```python
from build123d import *

# Parameters (mm, degrees)
F0_W     = 2
F0_H     = 4
F1_DEPTH = 8
F2_DEPTH = 9
F3_T     = -2
F4_R     = 5
F5_R     = 5
F6_W     = 8.62
F6_H     = 2
F7_DEPTH = 6


with BuildPart() as f1:
    # F0 (on Top) → F1 (new body)
    with BuildSketch(Plane.XY):
        Polygon((-23.121336045, 19.3491095896), (-19.6572344299, 21.3491095896), (-20.6572344299, 23.0811603972), (-24.121336045, 21.0811603972), align=None)
        Polygon((-7.4004464167, 26.1161683716), (-26.3174884677, 15.1944090512), (-26.3174884677, 10.3491095896), (-26.3174884677, 6.6491095896), (-26.3174884677, -15.1944090512), (-22.121336045, -17.617058782), (-18.917042051, -19.467058782), (0, -30.3888181024), (4.1961524227, -27.9661683716), (7.4004464167, -26.1161683716), (26.3174884677, -15.1944090512), (26.3174884677, -10.3491095896), (26.3174884677, -6.6491095896), (26.3174884677, 15.1944090512), (22.121336045, 17.617058782), (18.917042051, 19.467058782), (0, 30.3888181024), (-4.1961524227, 27.9661683716), align=None)
        Polygon((0, -21.59), (-18.6974884677, -10.795), (-18.6974884677, 10.795), (0, 21.59), (18.6974884677, 10.795), (18.6974884677, -10.795), align=None, mode=Mode.SUBTRACT)
        Polygon((-5.1961524227, -29.6982191792), (-8.6602540378, -27.6982191792), (-9.6602540378, -29.4302699868), (-6.1961524227, -31.4302699868), align=None)
        with Locations((29.3174884677, 8.3491095896)):
            Rectangle(F0_W, F0_H)
        with Locations((-29.3174884677, -8.3491095896)):
            Rectangle(F0_W, F0_H)
        Polygon((-26.3174884677, -15.1944090512), (-26.3174884677, 6.6491095896), (-28.3174884677, 6.6491095896), (-28.3174884677, -6.3491095896), (-28.3174884677, -10.3491095896), (-28.3174884677, -16.3491095896), (-23.121336045, -19.3491095896), (-22.121336045, -17.617058782), align=None)
        Polygon((-26.3174884677, 10.3491095896), (-26.3174884677, 15.1944090512), (-7.4004464167, 26.1161683716), (-8.4004464167, 27.8482191792), (-19.6572344299, 21.3491095896), (-23.121336045, 19.3491095896), (-28.3174884677, 16.3491095896), (-28.3174884677, 10.3491095896), align=None)
        Polygon((0, -30.3888181024), (-18.917042051, -19.467058782), (-19.917042051, -21.1991095896), (-8.6602540378, -27.6982191792), (-5.1961524227, -29.6982191792), (0, -32.6982191792), (5.1961524227, -29.6982191792), (4.1961524227, -27.9661683716), align=None)
        Polygon((28.3174884677, -10.3491095896), (26.3174884677, -10.3491095896), (26.3174884677, -15.1944090512), (7.4004464167, -26.1161683716), (8.4004464167, -27.8482191792), (19.6572344299, -21.3491095896), (23.121336045, -19.3491095896), (28.3174884677, -16.3491095896), align=None)
        Polygon((23.121336045, -19.3491095896), (19.6572344299, -21.3491095896), (20.6572344299, -23.0811603972), (24.121336045, -21.0811603972), align=None)
        Polygon((-5.1961524227, 29.6982191792), (-4.1961524227, 27.9661683716), (0, 30.3888181024), (18.917042051, 19.467058782), (19.917042051, 21.1991095896), (8.6602540378, 27.6982191792), (5.1961524227, 29.6982191792), (0, 32.6982191792), align=None)
        Polygon((6.1961524227, 31.4302699868), (5.1961524227, 29.6982191792), (8.6602540378, 27.6982191792), (9.6602540378, 29.4302699868), align=None)
        Polygon((23.121336045, 19.3491095896), (22.121336045, 17.617058782), (26.3174884677, 15.1944090512), (26.3174884677, -6.6491095896), (28.3174884677, -6.6491095896), (28.3174884677, 6.3491095896), (28.3174884677, 10.3491095896), (28.3174884677, 16.3491095896), align=None)
    extrude(amount=F1_DEPTH)

    # F0 (on Top) → F2 (join)
    with BuildSketch(Plane.XY):
        Polygon((-18.6974884677, 10.795), (-18.6974884677, -10.795), (0, -21.59), (18.6974884677, -10.795), (18.6974884677, 10.795), (0, 21.59), align=None)
    extrude(amount=F2_DEPTH)

    # F3: a shell. OpenCascade refuses it in one call, so the cavity is built on its own and cut out:
    # the body offset inwards by the wall thickness, plus a prism from it out through each open face.
    f3_core = offset(f1.part, amount=F3_T, kind=Kind.INTERSECTION, mode=Mode.PRIVATE)
    f3_exits = [f3_core.faces().sort_by_distance(p)[0] for p in [
        (0, 0, 2),
    ]]
    add(f3_core, mode=Mode.SUBTRACT)
    extrude(f3_exits, amount=-F3_T, mode=Mode.SUBTRACT)

    # F4
    f4_edges = [f1.edges().sort_by_distance(p)[0] for p in [
        (-18.697488, 10.795, 8.5),
        (-18.697488, -10.795, 8.5),
        (0, -21.59, 8.5),
        (18.697488, -10.795, 8.5),
        (18.697488, 10.795, 8.5),
        (0, 21.59, 8.5),
    ]]
    fillet(f4_edges, radius=F4_R)

    # F5
    f5_edges = [f1.edges().sort_by_distance(p)[0] for p in [
        (16.697488, -9.640299, 6.5),
        (0, -19.280599, 6.5),
        (-16.697488, -9.640299, 6.5),
        (-16.697488, 9.640299, 6.5),
        (0, 19.280599, 6.5),
        (16.697488, 9.640299, 6.5),
    ]]
    fillet(f5_edges, radius=F5_R)

    # F6 (on face) → F7 (join)
    with BuildSketch(Plane(origin=(0, 0, 6), x_dir=(1, 0, 0), z_dir=(0, 0, -1))):
        Polygon((15.2029661558, 21.6113814999), (13.4611243361, 22.6170343434), (8.3950167715, 15.6640247696), (10.0114517622, 14.4862565748), align=None)
        with Locations((-22.0074884677, 4.1833669636)):
            Rectangle(F6_W, F6_H)
        with Locations((22.0074884677, -0.0066501563)):
            Rectangle(F6_W, F6_H)
        Polygon((-12.5819755408, -13.1710924962), (-16.8919755408, -20.6362314769), (-15.1599247332, -21.6362314769), (-10.8499247332, -14.1710924962), align=None)
    extrude(amount=F7_DEPTH)


solid = f1.part
```
Geometry: final body of the model. Coordinates: model frame, mm. A direction names the side the tool comes from. Round coordinates to 2 decimals unless told otherwise and drop trailing zeros. Order: outer loops, then holes, each group sorted by start corner. A loop starts at its lowest first (then second) coordinate and runs counter-clockwise, first axis right, second up. Notation, with made-up numbers: (-20, 50.25) - (38, 50.25) arc R20 ccw to (38, 66.25) - close; hole circle Ø1 at (-4.75, -19). An arc over 180 degrees is marked (long way). Write item = value, one per line. Start each with the question number.
Q1. Cut plane A-A on y = 3. Return the cut outline in (x, z).
Q2. Access query for faces 4 (the flat face through (8.625, -24.238, 3.042)), 5 (the flat face through (20.54, 18.53, 3.94)), 6 (the flat face through (29, 6.349, 4)), 7 (the flat face through (-4.7, 28.84, 3.94)), 8 (the flat face through (-2.63, -31.18, 3.94)). Directions: +Z, -Z, +X, -X, +Y, -Y. A direction counts if a zero-diameter tool reaches every point of the face in a straight line with its end or side. Return the directions, or none.
Q3. Ray query, line 1 (X direction, y = 1.5, z = 6.75); line 2 (X direction, y = -15.5, z = 1.25); line 3 (X direction, y = -2.5, z = 4.5). Return the intervals inside material, ascending. Write a range as from..to.
Q4. Pull-direction query (Y, two-part tool) for faces 1 (the flat face through (22.365, -22.095, 3.944)), 2 (the flat face through (-23.36, -15.76, 3.04)), 3 (the flat face through (5.78, -27.05, 3.94)); classes: +Y half, -Y half, draft (parallel to the pull), parting line (faces both ways), or undercut.
Q5. Pin query (flat end, axial travel): pin 1 (0.6 mm diameter, centred on x = 25, z = 3, fed in from +Y); pin 2 (4 mm diameter, centred on y = 24.5, z = 1.5, fed in from -X); pin 3 (0.6 mm diameter, centred on x = 27.5, z = 3.5, fed in from +Y). Return the tip coordinate at first contact, or that it passes through.
Outcome:
q1.outline = (-28.32, 0) - (-26.32, 0) - (-26.32, 6) - (-16.7, 6) - (-16.7, 7) - (16.7, 7) - (16.7, 6) - (26.32, 6) - (26.32, 0) - (28.32, 0) - (28.32, 8) - (18.7, 8) - (18.7, 9) - (-18.7, 9) - (-18.7, 8) - (-28.32, 8) - close
q2.face_4 = -Z
q2.face_5 = +Z, -Z
q2.face_6 = +Z, -Z, +X, -Y
q2.face_7 = +Z, -Z, -X
q2.face_8 = +Z, -Z, -Y
q3.line_1 = -28.32..-16.7, 16.7..28.32
q3.line_2 = -28.32..-25.79, -23.21..-21.79, 8.62..10.75, 25.79..28.32
q3.line_3 = -28.32..-26.32, 26.32..28.32
q4.face_1 = -Y half
q4.face_2 = undercut
q4.face_3 = undercut
q5.pin_1 = 18.44
q5.pin_2 = -21.66
q5.pin_3 = 16.99
